from build123d import *

# Parameters (mm, degrees)
PAD_DEPTH       = 7.6
POCKET_DEPTH    = 6.6
SKETCH002_R     = 3
SKETCH002_R_2   = 1.5
PAD001_DEPTH    = 5
POCKET001_DEPTH = 2.5
SKETCH004_W     = 10
SKETCH004_H     = 2
PAD002_DEPTH    = 10
SKETCH005_R     = 1.5
POCKET002_DEPTH = 5


with BuildPart() as part:
    # Sketch → Pad (new body)
    with BuildSketch(Plane.XY):
        with BuildLine():
            Line((-27, 28), (27, 28))
            ThreePointArc((28, 27), (27.707107, 27.707107), (27, 28))
            Line((28, 27), (28, -27))
            ThreePointArc((27, -28), (27.707107, -27.707107), (28, -27))
            Line((27, -28), (-27, -28))
            ThreePointArc((-28, -27), (-27.707107, -27.707107), (-27, -28))
            Line((-28, -27), (-28, 27))
            ThreePointArc((-27, 28), (-27.707107, 27.707107), (-28, 27))
        make_face()
    extrude(amount=PAD_DEPTH)

    # Sketch001 (on Face10 of Pad) → Pocket (cut)
    with BuildSketch(Plane.XY.offset(7.6)):
        with BuildLine():
            Line((-25, 26), (25, 26))
            ThreePointArc((26, 25), (25.707107, 25.707107), (25, 26))
            Line((26, 25), (26, -25))
            ThreePointArc((25, -26), (25.707107, -25.707107), (26, -25))
            Line((25, -26), (-25, -26))
            ThreePointArc((-26, -25), (-25.707107, -25.707107), (-25, -26))
            Line((-26, -25), (-26, 25))
            ThreePointArc((-25, 26), (-25.707107, 25.707107), (-26, 25))
        make_face()
    extrude(amount=-POCKET_DEPTH, mode=Mode.SUBTRACT)

    # Sketch002 (on Face19 of Pocket) → Pad001 (join)
    with BuildSketch(Plane.XY.offset(1)):
        with Locations((-20.3447, -1.323)):
            Circle(SKETCH002_R)
        with Locations((-20.3447, -1.323)):
            Circle(SKETCH002_R_2, mode=Mode.SUBTRACT)
        with Locations((21.34, -21.243)):
            Circle(SKETCH002_R)
        with Locations((21.34, -21.243)):
            Circle(SKETCH002_R_2, mode=Mode.SUBTRACT)
    extrude(amount=PAD001_DEPTH)

    # Sketch003 (on Face5 of Pad001) → Pocket001 (cut)
    with BuildSketch(Plane.XY.offset(7.6)):
        Polygon((27.14591, 28.064611), (28.06645, 28.064611), (28.06645, -28.099016), (27.14591, -28.099016), (-28.144796, -28.099016), (-28.144796, -26.750607), (-28.144796, 28.064611), (-26.614367, 28.064611), align=None)
        with BuildLine():
            Line((27, -26), (27, 26))
            ThreePointArc((27, 26), (26.707107, 26.707107), (26, 27))
            Line((-26, 27), (26, 27))
            ThreePointArc((-26, 27), (-26.707107, 26.707107), (-27, 26))
            Line((-27, -26), (-27, 26))
            ThreePointArc((-27, -26), (-26.707107, -26.707107), (-26, -27))
            Line((-26, -27), (26, -27))
            ThreePointArc((26, -27), (26.707107, -26.707107), (27, -26))
        make_face(mode=Mode.SUBTRACT)
    extrude(amount=-POCKET001_DEPTH, mode=Mode.SUBTRACT)

    # Sketch004 (on Face6 of Pocket001) → Pad002 (join)
    with BuildSketch(Plane(origin=(0, 28, 0), x_dir=(-1, 0, 0), z_dir=(0, 1, 0))):
        with Locations((0, 1)):
            Rectangle(SKETCH004_W, SKETCH004_H)
    extrude(amount=PAD002_DEPTH)

    # Sketch005 (on Face21 of Pad002) → Pocket002 (cut)
    with BuildSketch(Plane.XY.offset(2)):
        with Locations((0, 34.384102)):
            Circle(SKETCH005_R)
        with BuildLine():
            Line((-3.5, 38), (3.5, 38))
            ThreePointArc((5, 36.5), (4.56066, 37.56066), (3.5, 38))
            Line((5, 36.5), (5, 28))
            Line((5.691499, 28), (5, 28))
            Line((5.691499, 38.719643), (5.691499, 28))
            Line((-5.537798, 38.719643), (5.691499, 38.719643))
            Line((-5.537798, 28), (-5.537798, 38.719643))
            Line((-5, 28), (-5.537798, 28))
            Line((-5, 36.5), (-5, 28))
            ThreePointArc((-3.5, 38), (-4.56066, 37.56066), (-5, 36.5))
        make_face()
    extrude(amount=-POCKET002_DEPTH, mode=Mode.SUBTRACT)


solid = part.part
Can you work these out from the model? Positions are in its coordinate system, mm. A direction names the side the tool comes from. Coordinates: 2 decimals unless noted, no trailing zeros. Order: outer loops, then holes, each group sorted by start corner. A loop starts at its lowest first (then second) coordinate and runs counter-clockwise, first axis right, second up. Notation, with made-up numbers: (85, -35.5) - (113, -35.5) arc R15 ccw to (113, -14.5) - close; hole circle Ø5 at (-2.75, -20). An arc over 180 degrees is marked (long way). Answer as a JSON object with one key per item and string values. Group by question number.
Q1. We'd pull the mould along Y, two halves only. Please class faces 5 (the face through (0, -28, 3)), 6 (the face through (-26, 0, 4)), 7 (the face through (-28, 0, 3)): +Y half, -Y half, draft (parallel to the pull), parting line (faces both ways), or undercut.
Q2. I need wall thicknesses on line 1 (Y direction, x = 0, z = 1.45); line 2 (Y direction, x = 21.34, z = 2.65); line 3 (Y direction, x = -1, z = 4.75). Which ranges of each line are inside material? Lowest first, please. Write a range as from..to.
Q3. Imagine slicing it at A-A (x = 0). Please give me the cut outline in (y, z).
Q4. Will these pins go through, and if not, where does the flat tip stop? P1, Ø3, axis at x = 13, y = 20, coming from the +Z side; P2, Ø0.6, axis at y = 34.5, z = 0.5, coming from the +X side; P3, Ø1.2, axis at y = 1.5, z = 6, coming from the -X side.
Q5. On a 3-axis mill with a long thin cutter (end or side, diameter ignored), from which of +Z, -Z, +X, -X, +Y, -Y can I reach the whole of each face in a straight line? I mean faces 1 (the face through (0, -2, 0)), 2 (the face through (26, 0, 4)), 3 (the face through (-5, 32, 1)), 4 (the face through (0, -27, 6)). Say none if no direction works.
Q6. Imagine slicing it at C-C (y = 12). Please give me the cut outline in (x, z).
Q7. Imagine slicing it at B-B (z = 4). Please give me the cut outline in (x, y), and give its area (3 significant figures).
Determined:
{
 "1": {"face 5": "-Y half", "face 6": "undercut", "face 7": "draft"},
 "2": {"line 1": "y = -28..-26, 26..32.88, 35.88..38", "line 2": "y = -28..-26, -24.24..-22.74, -19.74..-18.24, 26..28", "line 3": "y = -28..-26, 26..28"},
 "3": {"outline": "(-28, 0) - (32.88, 0) - (32.88, 2) - (28, 2) - (28, 5.1) - (27, 5.1) - (27, 7.6) - (26, 7.6) - (26, 1) - (-26, 1) - (-26, 7.6) - (-27, 7.6) - (-27, 5.1) - (-28, 5.1) - close; (35.88, 0) - (38, 0) - (38, 2) - (35.88, 2) - close"},
 "4": {"P1": "stops at z = 1", "P2": "stops at x = 5", "P3": "stops at x = -27"},
 "5": {"face 1": "-Z, +X, -X, +Y, -Y", "face 2": "+Z", "face 3": "+Z, -Z, -X, +Y", "face 4": "+Z, +X, -X, -Y"},
 "6": {"outline": "(-28, 0) - (28, 0) - (28, 5.1) - (27, 5.1) - (27, 7.6) - (26, 7.6) - (26, 1) - (-26, 1) - (-26, 7.6) - (-27, 7.6) - (-27, 5.1) - (-28, 5.1) - close"},
 "7": {"outline": "(-28, -27) arc R1 ccw to (-27, -28) - (27, -28) arc R1 ccw to (28, -27) - (28, 27) arc R1 ccw to (27, 28) - (-27, 28) arc R1 ccw to (-28, 27) - close; circle Ø6 at (-20.34, -1.32); circle Ø6 at (21.34, -21.24); hole (-26, -25) arc R1 ccw to (-25, -26) - (25, -26) arc R1 ccw to (26, -25) - (26, 25) arc R1 ccw to (25, 26) - (-25, 26) arc R1 ccw to (-26, 25) - close; hole circle Ø3 at (-20.34, -1.32); hole circle Ø3 at (21.34, -21.24)", "area": "474 mm2"}
}
